Source: CAD feature listing. Evaluate the final solid. Frame: model axes, mm. A direction names the side the tool comes from. Round coordinates to 2 decimals unless told otherwise and drop trailing zeros. Loops run counter-clockwise (first coordinate to the right, second up) from the corner with the lowest first, then second, coordinate; pieces in that order, holes last. Notation, with made-up numbers: (25.5, 66) -> (68.5, 66) arc R21 ccw to (68.5, 80) -> close; hole circle Ø6 at (-30.5, 62.5). An arc over 180 degrees is marked (long way). Return JSON: item names as keys, results as strings. Group by question number.
```python
from build123d import *
from OCP.BRepFilletAPI import BRepFilletAPI_MakeChamfer

# Parameters (mm, degrees)
BOSS_EXTRUDE2_DEPTH = 10
CHAMFER1_SIZE       = 5
CHAMFER1_SIZE2      = 1
CHAMFER2_SIZE       = 1
CHAMFER2_SIZE2      = 5


with BuildPart() as part:
    # Sketch2 → Boss-Extrude2 (new, symmetric)
    with BuildSketch(Plane.XY):
        Polygon((5.2, 3.3), (2.3, 6.2), (-2.3, 6.2), (-5.2, 3.3), (-5.2, 2.2), (-3, 2.2), (-3, -2.2), (-5.2, -2.2), (-5.2, -3.3), (-2.3, -6.2), (2.3, -6.2), (5.2, -3.3), (5.2, -2.2), (3, -2.2), (3, 2.2), (5.2, 2.2), align=None)
    extrude(amount=BOSS_EXTRUDE2_DEPTH, both=True)

    # Chamfer1: one chamfer whose edges measure the first distance from different faces: ONE call of the kernel's chamfer builder (chamfer() names one face for all edges)
    chamfer1_edges_1 = [part.edges().sort_by_distance(p)[0] for p in [
        (-3.75, 4.75, 10),
    ]]
    chamfer1_side_1 = [part.faces().sort_by_distance(p)[0] for p in [
        (-3.75, 4.75, 0),
    ]]
    chamfer1_edges_2 = [part.edges().sort_by_distance(p)[0] for p in [
        (3.75, 4.75, 10),
    ]]
    chamfer1_side_2 = [part.faces().sort_by_distance(p)[0] for p in [
        (3.75, 4.75, 0),
    ]]
    chamfer1_edges_3 = [part.edges().sort_by_distance(p)[0] for p in [
        (0, 6.2, 10),
    ]]
    chamfer1_side_3 = [part.faces().sort_by_distance(p)[0] for p in [
        (0, 6.2, 0),
    ]]
    chamfer1 = BRepFilletAPI_MakeChamfer(part.part.solid().wrapped)
    for e in chamfer1_edges_1:
        chamfer1.Add(CHAMFER1_SIZE, CHAMFER1_SIZE2, e.wrapped, chamfer1_side_1[0].wrapped)  # the first distance lies on this face
    for e in chamfer1_edges_2:
        chamfer1.Add(CHAMFER1_SIZE, CHAMFER1_SIZE2, e.wrapped, chamfer1_side_2[0].wrapped)  # the first distance lies on this face
    for e in chamfer1_edges_3:
        chamfer1.Add(CHAMFER1_SIZE, CHAMFER1_SIZE2, e.wrapped, chamfer1_side_3[0].wrapped)  # the first distance lies on this face
    add(Compound.cast(chamfer1.Shape()), mode=Mode.REPLACE)

    # Chamfer2
    chamfer2_edges = [part.edges().sort_by_distance(p)[0] for p in [
        (-3.75, 4.75, -10),
        (0, 6.2, -10),
        (3.75, 4.75, -10),
    ]]
    chamfer2_side = [part.faces().sort_by_distance(p)[0] for p in [
        (0, 0, -10),
    ]]
    chamfer(chamfer2_edges, length=CHAMFER2_SIZE, length2=CHAMFER2_SIZE2, reference=chamfer2_side[0])


solid = part.part
```
(1) Pin query (flat end, axial travel): pin 1 (3.5 mm diameter, centred on y = 0, z = -4.5, fed in from +X); pin 2 (2.5 mm diameter, centred on x = -4.5, z = -1.5, fed in from -Y); pin 3 (0.7 mm diameter, centred on x = -4.5, z = 1, fed in from +Y). Return the tip coordinate at first contact, or that it passes through.
(2) Ray query, line 1 (X direction, y = 2, z = -4.5); line 2 (Y direction, x = -3.5, z = 7.75); line 3 (Y direction, x = 4.5, z = 4). Return the intervals inside material, ascending.
(3) Cut plane B-B (z = 4.75). Return loops of the section in (x, y), and give its area (3 significant figures).
(4) Cut plane A-A (x = 1.5). Return loops of the section in (y, z).
(5) Set-up query: faces 1 (the face through (3, 0, 0)), 2 (the face through (-4, -2.2, 0)), 3 (the face through (-3.8, -4.7, 0.1)). Return all of +Z, -Z, +X, -X, +Y, -Y with unobstructed straight access to the full face (end or side cutting, diameter ignored); none if empty.
(6) Cut plane C-C (x = -3.75). Return loops of the section in (y, z), and give its area (3 significant figures).
(7) Mould query, pull axis Y, two halves, no side actions, for faces 4 (the face through (5.2, 3, 0)), 5 (the face through (0, 6.2, 0)), 6 (the face through (-3, 0, 0)), 7 (the face through (4, 2.2, 0)). Classes: released by +Y, released by -Y, zero draft, split by the parting line, or undercut.
(8) Cut plane D-D (y = -5). Return loops of the section in (x, z), and give its area (3 significant figures).
Answers follow:
{
 "1": {"pin 1": "x = 3", "pin 2": "y = -5.25", "pin 3": "y = 4.35"},
 "2": {"line 1": "-3 to 3", "line 2": "-5 to -2.2, 2.2 to 4.22", "line 3": "-4 to -2.2, 2.2 to 4"},
 "3": {"outline": "(-5.2, -3.3) -> (-2.3, -6.2) -> (2.3, -6.2) -> (5.2, -3.3) -> (5.2, -2.2) -> (3, -2.2) -> (3, 2.2) -> (5.2, 2.2) -> (5.2, 3.3) -> (2.3, 6.2) -> (-2.3, 6.2) -> (-5.2, 3.3) -> (-5.2, 2.2) -> (-3, 2.2) -> (-3, -2.2) -> (-5.2, -2.2) -> close", "area": "92.8 mm^2"},
 "4": {"outline": "(-6.2, -10) -> (5.2, -10) -> (6.2, -5) -> (6.2, 5) -> (5.2, 10) -> (-6.2, 10) -> close"},
 "5": {"face 1": "+Z, -Z, +X", "face 2": "+Z, -Z, -X", "face 3": "+Z, -Z, -X, -Y"},
 "6": {"outline": "(-4.75, -10) -> (-2.2, -10) -> (-2.2, 10) -> (-4.75, 10) -> close; (2.2, -10) -> (3.34, -10) -> (4.75, -5) -> (4.75, 5) -> (3.34, 10) -> (2.2, 10) -> close", "area": "94.9 mm^2"},
 "7": {"face 4": "zero draft", "face 5": "released by +Y", "face 6": "undercut", "face 7": "undercut"},
 "8": {"outline": "(-3.5, -10) -> (3.5, -10) -> (3.5, 10) -> (-3.5, 10) -> close", "area": "140 mm^2"}
}
